```python
from build123d import *

# Parameters (mm, degrees)
SKETCH1_W           = 120
SKETCH1_H           = 55
BOSS_EXTRUDE1_DEPTH = 5
SKETCH2_W           = 120
SKETCH2_H           = 7.5
BOSS_EXTRUDE2_DEPTH = 20
SKETCH3_W           = 120
SKETCH3_H           = 2.5
BOSS_EXTRUDE4_DEPTH = 20
BOSS_EXTRUDE5_DEPTH = 190
SKETCH9_W           = 310
SKETCH9_H           = 25
BOSS_EXTRUDE6_DEPTH = 70
SKETCH14_R          = 5.5
CUT_EXTRUDE5_DEPTH  = 153
SKETCH15_W          = 125
SKETCH15_H          = 25
CUT_EXTRUDE6_DEPTH  = 190
SKETCH16_W          = 120
SKETCH16_H          = 125
BOSS_EXTRUDE8_DEPTH = 10
SKETCH17_W          = 120
SKETCH17_H          = 125
CUT_EXTRUDE7_DEPTH  = 18
CUT_EXTRUDE8_START  = -18
SKETCH18_R          = 5.5
CUT_EXTRUDE8_DEPTH  = 18
CUT_EXTRUDE9_START  = -47
SKETCH20_R          = 5.483938487
SKETCH20_R_2        = 5.5
CUT_EXTRUDE9_DEPTH  = 47
CUT_EXTRUDE10_START = -47
SKETCH21_R          = 5.5
CUT_EXTRUDE10_DEPTH = 47
CUT_EXTRUDE11_START = -47
SKETCH22_R          = 5.5
CUT_EXTRUDE11_DEPTH = 47


with BuildPart() as part:
    # Sketch1 → Boss-Extrude1 (new body)
    with BuildSketch(Plane(origin=(0, 0, 0), x_dir=(1, 0, 0), z_dir=(0, 1, 0))):
        Rectangle(SKETCH1_W, SKETCH1_H)
    extrude(amount=BOSS_EXTRUDE1_DEPTH)

    # Sketch2 → Boss-Extrude2 (add)
    with BuildSketch(Plane(origin=(0, 5, 0), x_dir=(1, 0, 0), z_dir=(0, 1, 0))):
        with Locations((0, -23.75)):
            Rectangle(SKETCH2_W, SKETCH2_H)
    extrude(amount=BOSS_EXTRUDE2_DEPTH)

    # Sketch3 → Boss-Extrude4 (add)
    with BuildSketch(Plane(origin=(0, 5, 0), x_dir=(1, 0, 0), z_dir=(0, 1, 0))):
        with Locations((0, 26.25)):
            Rectangle(SKETCH3_W, SKETCH3_H)
    extrude(amount=BOSS_EXTRUDE4_DEPTH)

    # Sketch8 → Boss-Extrude5 (add)
    with BuildSketch(Plane.ZY.offset(60)):
        Polygon((-27.5, 0), (-27.5, 25), (-25, 25), (-25, 5), (20, 5), (20, 25), (27.5, 25), (27.5, 0), align=None)
    extrude(amount=BOSS_EXTRUDE5_DEPTH)

    # Sketch9 → Boss-Extrude6 (add)
    with BuildSketch(Plane(origin=(0, 0, -27.5), x_dir=(-1, 0, 0), z_dir=(0, 0, -1))):
        with Locations((95, 12.5)):
            Rectangle(SKETCH9_W, SKETCH9_H)
    extrude(amount=BOSS_EXTRUDE6_DEPTH)

    # Sketch14 → Cut-Extrude5 (cut)
    with BuildSketch(Plane(origin=(0, 0, 0), x_dir=(-1, 0, 0), z_dir=(0, -1, 0))):
        with Locations(Location((225.445279058, 7.255161462, 0), (0, 0, 90))):
            Circle(SKETCH14_R)
        with Locations(Location((175.445279058, 7.255161462, 0), (0, 0, 90))):
            Circle(SKETCH14_R)
        with Locations(Location((225.445279058, 57.255161462, 0), (0, 0, 90))):
            Circle(SKETCH14_R)
        with Locations(Location((148.0182107, 48.5, 0), (0, 0, 90))):
            Circle(SKETCH14_R)
        with Locations(Location((183.240850763, 83.987541856, 0), (0, 0, 90))):
            Circle(SKETCH14_R)
    extrude(amount=-CUT_EXTRUDE5_DEPTH, mode=Mode.SUBTRACT)

    # Sketch15 → Cut-Extrude6 (cut)
    with BuildSketch(Plane(origin=(60, 0, 0), x_dir=(0, 0, -1), z_dir=(1, 0, 0))):
        with Locations((35, 12.5)):
            Rectangle(SKETCH15_W, SKETCH15_H)
    extrude(amount=-CUT_EXTRUDE6_DEPTH, mode=Mode.SUBTRACT)

    # Sketch16 → Boss-Extrude8 (add)
    with BuildSketch(Plane(origin=(0, 0, 0), x_dir=(-1, 0, 0), z_dir=(0, -1, 0))):
        with Locations((190, 35)):
            Rectangle(SKETCH16_W, SKETCH16_H)
    extrude(amount=BOSS_EXTRUDE8_DEPTH)

    # Sketch17 → Cut-Extrude7 (cut)
    with BuildSketch(Plane(origin=(0, 25, 0), x_dir=(1, 0, 0), z_dir=(0, 1, 0))):
        with Locations((-190, 35)):
            Rectangle(SKETCH17_W, SKETCH17_H)
    extrude(amount=-CUT_EXTRUDE7_DEPTH, mode=Mode.SUBTRACT)

    # Sketch18 → Cut-Extrude8 (cut)
    with BuildSketch(Plane(origin=(0, 7, 0), x_dir=(1, 0, 0), z_dir=(0, 1, 0)).offset(CUT_EXTRUDE8_START)):
        with Locations(Location((-148.0182107, 48.5, 0), (0, 0, 270))):
            Circle(SKETCH18_R)
    extrude(amount=CUT_EXTRUDE8_DEPTH, mode=Mode.SUBTRACT)

    # Sketch20 → Cut-Extrude9 (cut)
    with BuildSketch(Plane(origin=(0, 7, 0), x_dir=(1, 0, 0), z_dir=(0, 1, 0)).offset(CUT_EXTRUDE9_START)):
        with Locations(Location((-183.240850763, 83.987541856, 0), (0, 0, 270))):
            Circle(SKETCH20_R)
        with Locations(Location((-225.445279058, 57.255161462, 0), (0, 0, 270))):
            Circle(SKETCH20_R_2)
    extrude(amount=CUT_EXTRUDE9_DEPTH, mode=Mode.SUBTRACT)

    # Sketch21 → Cut-Extrude10 (cut)
    with BuildSketch(Plane(origin=(0, 5, 0), x_dir=(1, 0, 0), z_dir=(0, 1, 0)).offset(CUT_EXTRUDE10_START)):
        with Locations(Location((-225.445279058, 7.255161462, 0), (0, 0, 90))):
            Circle(SKETCH21_R)
    extrude(amount=CUT_EXTRUDE10_DEPTH, mode=Mode.SUBTRACT)

    # Sketch22 → Cut-Extrude11 (cut)
    with BuildSketch(Plane(origin=(0, 5, 0), x_dir=(1, 0, 0), z_dir=(0, 1, 0)).offset(CUT_EXTRUDE11_START)):
        with Locations(Location((-175.445279058, 7.255161462, 0), (0, 0, 90))):
            Circle(SKETCH22_R)
    extrude(amount=CUT_EXTRUDE11_DEPTH, mode=Mode.SUBTRACT)


solid = part.part
```
Design review of the part built by this model. Coordinates are the model's own, in mm. A direction names the side the tool comes from. Coordinates: 2 decimals unless noted, no trailing zeros. Order: outer loops, then holes, each group sorted by start corner. A loop starts at its lowest first (then second) coordinate and runs counter-clockwise, first axis right, second up.
1) Take a section at A-A, the plane z = -48.5. Give the boundary of the cut face in (x, y).
2) Take a section at B-B, the plane y = 3. Give the boundary of the cut face in (x, z).
3) Mouldability with a two-part tool opening along X and no side actions: class faces 1 (the flat face through (-250, -1, -34)), 2 (the cylindrical face through (-188.106, -5.07, -81.457)), 3 (the flat face through (-189, -10, -36)) as +X half, -X half, draft (parallel to the pull), parting line (faces both ways), or undercut.
4) Clearance check with a flat-ended pin moving along its axis: pin 1 (13.5 mm diameter, centred on x = -168, z = -4, fed in from +Y). State where the tip first meets the part, or that it passes through.
5) Take a section at D-D, the plane x = -227. Give the boundary of the cut face in (y, z), and give its area (3 significant figures).
6) Take a section at C-C, the plane x = -152. Give the boundary of the cut face in (y, z).
7) Wall thickness on line 1 along Z through (x, y) = (-197.5, 6); line 2 along X through (y, z) = (2.25, -10); line 3 along X through (y, z) = (-2.25, -48.5): over which ranges is each line inside the solid? List them lowest first.
8) For faces 4 (the cylindrical face through (-180.814, -2.605, -6.063)), 5 (the flat face through (-189, 5, -3)), list the 3-axis set-ups (+Z, -Z, +X, -X, +Y, -Y) from which the entire face can be reached by the end or side of a thin tool; tool diameter is ignored.
Returned:
1. outline: (-250, -10) - (-153.52, -10) - (-153.52, 7) - (-250, 7) - close; (-142.52, -10) - (-130, -10) - (-130, 7) - (-142.52, 7) - close
2. outline: (-250, -97.5) - (-130, -97.5) - (-130, 27.5) - (-250, 27.5) - close; hole circle Ø11 at (-225.45, -57.26); hole circle Ø11 at (-225.45, -7.26); hole circle Ø11 at (-183.24, -83.99); hole circle Ø11 at (-175.45, -7.26); hole circle Ø11 at (-148.02, -48.5)
3. face 1: -X half
3. face 2: undercut
3. face 3: draft
4. pin 1: stops at y = 5
5. outline: (-10, -97.5) - (7, -97.5) - (7, -62.53) - (-10, -62.53) - close; (-10, -51.98) - (7, -51.98) - (7, -25) - (5, -25) - (5, -12.53) - (-10, -12.53) - close; (-10, -1.98) - (5, -1.98) - (5, 20) - (7, 20) - (7, 27.5) - (-10, 27.5) - close
5. area: 1,700 mm2
6. outline: (-10, -97.5) - (7, -97.5) - (7, -52.29) - (-10, -52.29) - close; (-10, -44.71) - (7, -44.71) - (7, -25) - (5, -25) - (5, 20) - (7, 20) - (7, 27.5) - (-10, 27.5) - close
7. line 1: z = -97.5 to -25, 20 to 27.5
7. line 2: x = -250 to -230.21, -220.68 to -180.21, -170.68 to -130
7. line 3: x = -250 to -153.52, -142.52 to -130
8. face 4: +Y, -Y
8. face 5: +X, -X, +Y
